```python
from build123d import *

# Parameters (mm, degrees)
SKETCH1_W           = 300
SKETCH1_H           = 200
BOSS_EXTRUDE1_DEPTH = 10
SKETCH2_R           = 5
SKETCH2_W           = 90
SKETCH2_H           = 10
BOSS_EXTRUDE2_DEPTH = 10


with BuildPart() as part:
    # Sketch1 → Boss-Extrude1 (new body)
    with BuildSketch(Plane(origin=(0, 0, 0), x_dir=(1, 0, 0), z_dir=(0, 1, 0))):
        with Locations((150, 100)):
            Rectangle(SKETCH1_W, SKETCH1_H)
    extrude(amount=BOSS_EXTRUDE1_DEPTH)

    # Sketch2 → Boss-Extrude2 (add)
    with BuildSketch(Plane(origin=(0, 10, 0), x_dir=(1, 0, 0), z_dir=(0, 1, 0))):
        with Locations((30, 100)):
            Circle(SKETCH2_R)
        with Locations((105, 115)):
            Rectangle(SKETCH2_W, SKETCH2_H)
        with Locations((105, 85)):
            Rectangle(SKETCH2_W, SKETCH2_H)
    extrude(amount=BOSS_EXTRUDE2_DEPTH)


solid = part.part
```
Design review of the part built by this model. Coordinates are the model's own, in mm. A direction names the side the tool comes from. Give positions to 0.01 mm unless a question says otherwise; leave off trailing zeros. Loops run counter-clockwise (first coordinate to the right, second up) from the corner with the lowest first, then second, coordinate; pieces in that order, holes last. Notation, with made-up numbers: (58.5, 64.25) -> (63.5, 64.25) arc R4 cw to (63.5, 68.25) -> close; hole circle Ø11 at (19, 88). An arc over 180 degrees is marked (long way). Write each question's results on one line, items separated by ' | '.
Q1. Wall thickness on L1, parallel to Z at x = 93, y = 12.75; L2, parallel to Y at x = 116.5, z = -126; L3, parallel to X at y = 12.25, z = -118.5: over which ranges is each line inside the solid? List them lowest first.
Reply:
L1: z = -120 to -110, -90 to -80 | L2: y = 0 to 10 | L3: x = 60 to 150
Q2. Take a section at D-D, the plane x = 30. Write out the cut boundary in (y, z), plus the area to 3 significant figures.
Reply:
outline: (0, -200) -> (10, -200) -> (10, -105) -> (20, -105) -> (20, -95) -> (10, -95) -> (10, 0) -> (0, 0) -> close | area: 2,100 mm²
Q3. Take a section at B-B, the plane x = 144. Write out the cut boundary in (y, z).
Reply:
outline: (0, -200) -> (10, -200) -> (10, -120) -> (20, -120) -> (20, -110) -> (10, -110) -> (10, -90) -> (20, -90) -> (20, -80) -> (10, -80) -> (10, 0) -> (0, 0) -> close
Q4. For pin 1 Ø5 at (y, z) = (17, -117) entering from +X; pin 2 Ø3 at (y, z) = (14, -83.5) entering from -X; pin 3 Ø8 at (x, z) = (176.5, -129) entering from +Y, all flat-tipped, find the tip position at first contact; note any pin that passes through.
Reply:
pin 1: stops at x = 150 | pin 2: stops at x = 60 | pin 3: stops at y = 10
Q5. Machinability: for faces 1 (the face through (104, 15, -120)), 2 (the face through (150, 15, -85)), 3 (the face through (60, 15, -115)), 4 (the face through (104, 15, -80)), which of the approach directions +Z, -Z, +X, -X, +Y, -Y give a long, thin tool a straight path to every point of the face, cutting with its end or side? Answer none if there is none.
Reply:
face 1: -Z, +X, -X, +Y | face 2: +Z, -Z, +X, +Y | face 3: +Z, -Z, -X, +Y | face 4: +Z, +X, -X, +Y
Q6. The part is to be moulded in two halves that separate along Z. For faces 5 (the face through (104, 15, -110)), 6 (the face through (150, 15, -115)), 7 (the face through (25, 15, -100)), say which applies: +Z half, -Z half, draft (parallel to the pull), parting line (faces both ways), or undercut.
Reply:
face 5: undercut | face 6: draft | face 7: parting line
Q7. Take a section at C-C, the plane z = -100. Write out the cut boundary in (x, y).
Reply:
outline: (0, 0) -> (300, 0) -> (300, 10) -> (35, 10) -> (35, 20) -> (25, 20) -> (25, 10) -> (0, 10) -> close
Q8. Take a section at A-A, the plane y = 13.5. Write out the cut boundary in (x, z).
Reply:
outline: circle Ø10 at (30, -100); (60, -120) -> (150, -120) -> (150, -110) -> (60, -110) -> close; (60, -90) -> (150, -90) -> (150, -80) -> (60, -80) -> close
